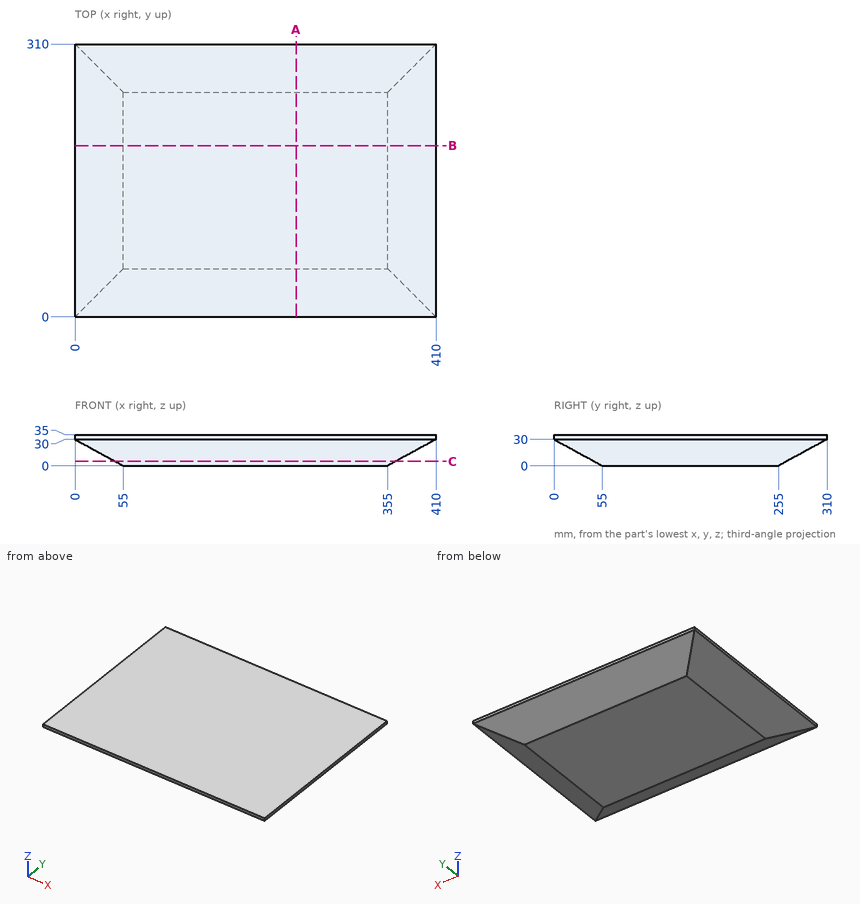
Can you work these out from the drawing? Everything is in mm from the part's minimum corner. Coordinates: 2 decimals unless noted, no trailing zeros. Write each loop counter-clockwise with the first axis right and the second up, starting at its lowest first coordinate (ties: lowest second). Pieces come first, ordered by that corner, then holes. Notation, with made-up numbers: (-23, 31.5) -> (32, 31.5) arc R8 ccw to (32, 38.5) -> close; hole circle Ø9 at (69.5, 46.25). An arc over 180 degrees is marked (long way). Write each question's results on one line, items separated by ' | '. Start each with the question number.
Item 1: If we section it at C-C, the plane z = 5: Write out the boundary of the cut face in (x, y), and give its area (3 significant figures).
Item 2: Please list where these lines run through material, in increasing order: probe 1 along X at (y, z) = (129, 5.5); probe 2 along Z at (x, y) = (198.5, 21); probe 3 along X at (y, z) = (106, 23).
Item 3: If we section it at B-B, the plane y = 194.5: Write out the boundary of the cut face in (x, z), and give its area (3 significant figures).
Item 4: I'm going to push flat-ended pins straight in: P1, Ø10, axis at x = 55, z = 18.5, coming from the -Y side; P2, Ø5, axis at x = 255, z = 20, coming from the +Y side; P3, Ø1.5, axis at x = 201, z = 22, coming from the -Y side. Where does each tip first touch, or does it pass through?
Item 5: If we section it at A-A, the plane x = 251: Write out the boundary of the cut face in (y, z).
Answer block:
1) outline: (45.83, 45.83) -> (364.17, 45.83) -> (364.17, 264.17) -> (45.83, 264.17) -> close | area: 69,500 mm²
2) probe 1: 44.92 to 365.08 | probe 2: 18.55 to 35 | probe 3: 12.83 to 397.17
3) outline: (0, 30) -> (55, 0) -> (355, 0) -> (410, 30) -> (410, 35) -> (0, 35) -> close | area: 12,700 mm²
4) P1: y = 11.92 | P2: y = 296.25 | P3: y = 13.29
5) outline: (0, 30) -> (55, 0) -> (255, 0) -> (310, 30) -> (310, 35) -> (0, 35) -> close
